Could you check a few things on this model? Use its own coordinates, in mm. A direction names the side the tool comes from. Give positions to 0.01 mm unless a question says otherwise; leave off trailing zeros. Order: outer loops, then holes, each group sorted by start corner. A loop starts at its lowest first (then second) coordinate and runs counter-clockwise, first axis right, second up. Notation, with made-up numbers: M 65,13.25 L 118,13.25 A16 ccw 118,41.25 Z; hole C 67,56.25 d6. An arc over 180 degrees is marked long. Use a Markdown table: item, result. Add a question column.
Item 1: I'm going to push flat-ended pins straight in: pin 1 Ø2 at (x, y) = (18.5, -15) entering from +Z; pin 2 Ø3 at (y, z) = (-15, 7.5) entering from -X; pin 3 Ø1 at (x, z) = (14, 21.5) entering from -Y; pin 4 Ø5 at (x, z) = (49.5, 18.5) entering from +Y. Where does each tip first touch, or does it pass through?
Item 2: Suppose I cut it at D-D on y = -7. Write out the boundary of the cut face in (x, z).
Item 3: For faces 4 (the face through (63.7, -6.3, 37.9)), 5 (the face through (57.15, -43, 5)), 6 (the face through (11, -23, 11)), which set-ups out of +Z, -Z, +X, -X, +Y, -Y let a thin tool reach every point of the face, with its end or its side?
Item 4: If we mould it in two halves opening along X, with no side actions, what happens to faces 1 (the face through (29, -12.7, 31)), 2 (the face through (19.05, -43, 5)), 3 (the face through (61.7, -27.1, 14.5))? For each: released by +X, released by -X, zero draft, split by the parting line, or undercut.
Item 5: Suppose I cut it at C-C on x = 39. Write out the boundary of the cut face in (y, z), plus the area to 3 significant figures.
Item 6: Suppose I cut it at A-A on y = -39. Write out the boundary of the cut face in (x, z).
Item 7: Suppose I cut it at B-B on z = 6. Write out the boundary of the cut face in (x, y), plus the area to 3 significant figures.
Item 8: If I drill on L1, parallel to Y at x = 42, z = 34.5; L2, parallel to X at y = -38.5, z = 11; L3, parallel to Z at x = 38.5, y = -33.5, over which ranges is the centre line in solid material (lowest first)? Write a range as from..to.
from build123d import *

# Parameters (mm, degrees)
F1_DEPTH = 12.7
F3_DEPTH = 38.1
F4_W     = 38.1
F4_H     = 12.7
F5_DEPTH = 50.801
F7_DEPTH = 76.201


with BuildPart() as f1:
    # F0 (on Front) → F1 (new body)
    with BuildSketch(Plane.XZ):
        Polygon((25.4, 50.8), (0, 25.4), (0, 0), (76.2, 0), (76.2, 25.4), (50.8, 50.8), align=None)
    extrude(amount=F1_DEPTH)

    # F2 (on face) → F3 (join)
    with BuildSketch(Plane.XZ.offset(12.7)):
        Polygon((0, 0), (76.2, 0), (38.1, 38.1), align=None)
    extrude(amount=F3_DEPTH)

    # F4 (on face) → F5 (cut, through all)
    with BuildSketch(Plane(origin=(0, 0, 0), x_dir=(1, 0, 0), z_dir=(0, 0, -1))):
        with Locations((38.1, 44.45)):
            Rectangle(F4_W, F4_H)
    extrude(amount=-F5_DEPTH, mode=Mode.SUBTRACT)

    # F6 (on face) → F7 (cut, through all)
    with BuildSketch(Plane.YZ.offset(76.2)):
        Polygon((-51.202006, -0.734927), (-12.7, 38.1), (-51.202006, 38.1), align=None)
    extrude(amount=-F7_DEPTH, mode=Mode.SUBTRACT)


solid = f1.part
Findings below:
| question | item | result |
|---|---|---|
| 1 | pin 1 | stops at z = 19.5 |
| 1 | pin 2 | stops at x = 6 |
| 1 | pin 3 | stops at y = -12.7 |
| 1 | pin 4 | stops at y = 0 |
| 2 | outline | M 0,0 L 76.2,0 L 76.2,25.4 L 50.8,50.8 L 25.4,50.8 L 0,25.4 Z |
| 3 | face 4 | +Z, +X, +Y, -Y |
| 3 | face 5 | +Z, -Z, -Y |
| 3 | face 6 | +Z, -X, -Y |
| 4 | face 1 | zero draft |
| 4 | face 2 | undercut |
| 4 | face 3 | released by +X |
| 5 | outline | M -38.1,0 L 0,0 L 0,50.8 L -12.7,50.8 L -12.7,37.2 L -13.59,37.2 L -38.1,12.48 Z |
| 5 | area | 1,290 mm^2 |
| 6 | outline | M 0,0 L 19.05,0 L 19.05,11.57 L 11.57,11.57 Z; M 57.15,0 L 76.2,0 L 64.63,11.57 L 57.15,11.57 Z |
| 7 | outline | M 0,-12.7 L 6,-12.7 L 6,-44.52 L 19.05,-44.52 L 19.05,-38.1 L 57.15,-38.1 L 57.15,-44.52 L 70.2,-44.52 L 70.2,-12.7 L 76.2,-12.7 L 76.2,0 L 0,0 Z |
| 7 | area | 2,770 mm^2 |
| 8 | L1 | y = -12.7..0 |
| 8 | L2 | x = 11..19.05, 57.15..65.2 |
| 8 | L3 | z = 0..17.12 |
